from build123d import *

# Parameters (mm, degrees)
SKETCH_1_W          = 9.03
SKETCH_1_H          = 11.2
EXTRUDE_1_DEPTH     = 4.38
FILLET_1_R          = 0.5
CUT_EXTRUDE_2_DEPTH = 14.38
FILLET_5_R          = 2
FILLET_6_R          = 1
FILLET_7_R          = 0.5


with BuildPart() as part:
    # 스케치1 → 보스-돌출1 (new body)
    with BuildSketch(Plane.XY):
        Rectangle(SKETCH_1_W, SKETCH_1_H)
    extrude(amount=EXTRUDE_1_DEPTH)

    # 필렛1
    fillet_1_edges = [part.edges().sort_by_distance(p)[0] for p in [
        (-4.515, 0, 0),
        (4.515, 0, 0),
    ]]
    fillet(fillet_1_edges, radius=FILLET_1_R)

    # 스케치2 → 컷-돌출2 (cut)
    with BuildSketch(Plane(origin=(0, 5.6, 0), x_dir=(1, 0, 0), z_dir=(0, 1, 0))):
        Polygon((4.165, -4.03), (4.165, -0.35), (-4.165, -0.35), (-4.165, -4.03), (-2.5, -4.03), (0, -2.19), (2.5, -4.03), align=None)
        Polygon((2.5, -4.38), (2.024456522, -4.03), (-2.024456522, -4.03), (-2.5, -4.38), align=None)
        Polygon((-2.024456522, -4.03), (2.024456522, -4.03), (0, -2.54), align=None)
    extrude(amount=-CUT_EXTRUDE_2_DEPTH, mode=Mode.SUBTRACT)

    # 필렛5
    # the kernel refuses this fillet: 2 mm, written as the material it adds along each edge
    with BuildSketch(Plane(origin=(4.165, 5.6, 4.03), x_dir=(-1, 0, 0), z_dir=(0, -1, 0))) as fillet_5_piece_1:
        with BuildLine():
            CenterArc((2, 1.971744152), FILLET_5_R, 180, 80.357504536)
            Line((0, 1.971744152), (0, 0))
            Line((0, 0), (1.665, 0))
        make_face()
    extrude(amount=11.2)
    with BuildSketch(Plane(origin=(-4.165, 5.6, 4.03), x_dir=(0, 0, -1), z_dir=(0, -1, 0))) as fillet_5_piece_2:
        with BuildLine():
            CenterArc((1.971744152, 2), FILLET_5_R, 189.642495464, 80.357504536)
            Line((0, 1.665), (0, 0))
            Line((0, 0), (1.971744152, 0))
        make_face()
    extrude(amount=11.2)
    # the kernel refuses this fillet: 2 mm, written as the material it takes off along each edge
    with BuildSketch(Plane(origin=(4.515, -10.6, 4.38), x_dir=(0, 0, -1), z_dir=(0, 1, 0))) as fillet_5_2_piece_1:
        with BuildLine():
            CenterArc((FILLET_5_R, FILLET_5_R), FILLET_5_R, 180, 90)
            Line((0, FILLET_5_R), (0, 0))
            Line((0, 0), (FILLET_5_R, 0))
        make_face()
    extrude(amount=21.2, mode=Mode.SUBTRACT)
    with BuildSketch(Plane(origin=(-4.515, 10.6, 4.38), x_dir=(1, 0, 0), z_dir=(0, -1, 0))) as fillet_5_2_piece_2:
        with BuildLine():
            CenterArc((FILLET_5_R, -FILLET_5_R), FILLET_5_R, 90, 90)
            Line((0, -FILLET_5_R), (0, 0))
            Line((0, 0), (FILLET_5_R, 0))
        make_face()
    extrude(amount=21.2, mode=Mode.SUBTRACT)

    # 필렛6
    fillet_6_edges = [part.edges().sort_by_distance(p)[0] for p in [
        (2.5, 0, 4.03),
        (2.5, 0, 4.38),
        (-2.5, 0, 4.38),
        (-2.5, 0, 4.03),
    ]]
    fillet(fillet_6_edges, radius=FILLET_6_R)

    # 필렛7
    fillet_7_edges = [part.edges().sort_by_distance(p)[0] for p in [
        (-4.165, 0, 0.35),
        (4.165, 0, 0.35),
    ]]
    fillet(fillet_7_edges, radius=FILLET_7_R)


solid = part.part
Geometry check sheet. Reference: the model listing, model coordinates, mm. A direction names the side the tool comes from. Give positions to 0.01 mm unless a question says otherwise; leave off trailing zeros. Order: outer loops, then holes, each group sorted by start corner. A loop starts at its lowest first (then second) coordinate and runs counter-clockwise, first axis right, second up.
1. Sectioned sample at B-B (x = -0.75). Record the boundary of the cut face in (y, z).
Completed:
outline: (-5.6, 0) - (5.6, 0) - (5.6, 0.35) - (-5.6, 0.35) - close; (-5.6, 2.74) - (5.6, 2.74) - (5.6, 3.09) - (-5.6, 3.09) - close
2. Access from +Z, -Z, +X, -X, +Y, -Y to the whole of each face (thin tool, end or side, straight path). Record for faces 1 (the face through (2.619, -0.078, 3.916)), 2 (the face through (4.515, 0, 1)).
Completed:
face 1: +Y, -Y
face 2: +Z, -Z, +X, +Y, -Y
3. Sectioned sample at A-A (z = 1.8). Record the boundary of the cut face in (x, y) (3 decimals).
Completed:
outline: (-4.515, -5.6) - (-4.165, -5.6) - (-4.165, 5.6) - (-4.515, 5.6) - close; (4.165, -5.6) - (4.515, -5.6) - (4.515, 5.6) - (4.165, 5.6) - close
4. Draft check along Z on faces 3 (the face through (4.165, 0, 1)), 4 (the face through (-4.515, 0, 1)), 5 (the face through (4.1, -0.1, 3.6)), 6 (the face through (0, 0, 0)). Enter one of: pulls with the +Z half, pulls with the -Z half, needs draft (parallel to the pull), parting line crosses it, or undercut.
Completed:
face 3: undercut
face 4: needs draft
face 5: pulls with the +Z half
face 6: pulls with the -Z half
5. Depth check by flat-ended pin: pin 1 (2 mm diameter, centred on y = -2, z = 3, fed in from -X) (3 decimals). Enter the tip coordinate at first touch or a pass-through.
Completed:
pin 1: stops at x = -4.515
6. Scan lines: line 1 (Z direction, x = 2, y = 2); line 2 (X direction, y = -4, z = 3.2); line 3 (X direction, y = 4.75, z = 2.25) (3 decimals). Record each from-to range of solid material in increasing order.
Completed:
line 1: z = 0 to 0.35, 3.66 to 4.01
line 2: x = -4.34 to -3.81, -1.37 to -0.9, 0.9 to 1.37, 3.81 to 4.34
line 3: x = -4.515 to -4.156, -0.082 to 0.082, 4.156 to 4.515
